Geometry: final body of the model. Coordinates: model frame, mm. A direction names the side the tool comes from. Round coordinates to 2 decimals unless told otherwise and drop trailing zeros. Write each loop counter-clockwise with the first axis right and the second up, starting at its lowest first coordinate (ties: lowest second). Pieces come first, ordered by that corner, then holes.
from build123d import *

# Parameters (mm, degrees)
ESQUISSE1_W             = 165.35
ESQUISSE1_H             = 84.146
BOSS_EXTRU_1_DEPTH      = 3.175
ESQUISSE2_W             = 3.175
ESQUISSE2_H             = 32.073
ENL_V_MAT_EXTRU_1_DEPTH = 93.819036727
ESQUISSE3_W             = 20
ESQUISSE3_H             = 3.175
ENL_V_MAT_EXTRU_2_DEPTH = 93.819036727


with BuildPart() as part:
    # Esquisse1 → Boss.-Extru.1 (new body)
    with BuildSketch(Plane.XY):
        Rectangle(ESQUISSE1_W, ESQUISSE1_H)
    extrude(amount=BOSS_EXTRU_1_DEPTH)

    # Esquisse2 → Enlèv. mat.-Extru.1 (cut, through all)
    with BuildSketch(Plane.XY.offset(3.175)):
        with Locations((-81.0875, -26.0365)):
            Rectangle(ESQUISSE2_W, ESQUISSE2_H)
        with Locations((-81.0875, 26.0365)):
            Rectangle(ESQUISSE2_W, ESQUISSE2_H)
    enl_v_mat_extru_1 = extrude(amount=-ENL_V_MAT_EXTRU_1_DEPTH, mode=Mode.SUBTRACT)

    # Symétrie1: Enlèv. mat.-Extru.1 across plane
    add(enl_v_mat_extru_1.mirror(Plane(origin=(0, 0, 0), x_dir=(0, 0, 1), z_dir=(1, 0, 0))), mode=Mode.SUBTRACT)

    # Esquisse3 → Enlèv. mat.-Extru.2 (cut, through all)
    with BuildSketch(Plane.XY.offset(3.175)):
        with Locations((0, -40.4855)):
            Rectangle(ESQUISSE3_W, ESQUISSE3_H)
        with Locations((40, -40.4855)):
            Rectangle(ESQUISSE3_W, ESQUISSE3_H)
        with Locations((-40, -40.4855)):
            Rectangle(ESQUISSE3_W, ESQUISSE3_H)
    enl_v_mat_extru_2 = extrude(amount=-ENL_V_MAT_EXTRU_2_DEPTH, mode=Mode.SUBTRACT)

    # Symétrie2: Enlèv. mat.-Extru.2 across plane
    add(enl_v_mat_extru_2.mirror(Plane.ZX), mode=Mode.SUBTRACT)


solid = part.part
1) Draft query along X for faces 4 (the flat face through (20, -42.073, 2)), 5 (the flat face through (-82.675, 0, 2)), 6 (the flat face through (-50, -41, 2)). Return one class per face: pulls with the +X half, pulls with the -X half, needs draft (parallel to the pull), parting line crosses it, or undercut.
2) First-contact query: P1, Ø1, axis at x = -40.5, y = -23, coming from the -Z side; P2, Ø1, axis at x = -44, z = 1, coming from the +Y side; P3, Ø1, axis at x = 36.5, z = 2, coming from the -Y side; P4, Ø1.6, axis at y = -40.5, z = 2, coming from the +X side. Flat tips, straight axial feed; report the tip coordinate or a pass-through.
3) Reachability of faces 1 (the flat face through (-40, 38.898, 2)), 2 (the flat face through (-79.5, 26, 2)), 3 (the flat face through (10, -41, 2)) from +Z, -Z, +X, -X, +Y, -Y: full face, straight path, thin tool, end or side. Return the list, or none.
4) Section A-A on y = -34. Output: boundary loops of the cut face in (x, z) (3 decimals), plus the area to 3 significant figures.
5) Line query: probe 1 along Y at (x, z) = (30.5, 2); probe 2 along X at (y, z) = (17.5, 0.7). Output: solid intervals per line, ascending.
6) Section B-B on x = 3. Output: boundary loops of the cut face in (y, z) (3 decimals).
Filled in:
1. face 4: needs draft
1. face 5: pulls with the -X half
1. face 6: undercut
2. P1: stops at z = 0
2. P2: stops at y = 38.9
2. P3: stops at y = -38.9
2. P4: stops at x = 79.5
3. face 1: +Z, -Z, +Y
3. face 2: +Z, -Z, -X, +Y
3. face 3: +Z, -Z, -Y
4. outline: (-79.5, 0) - (79.5, 0) - (79.5, 3.175) - (-79.5, 3.175) - close
4. area: 505 mm2
5. probe 1: y = -38.9 to 38.9
5. probe 2: x = -79.5 to 79.5
6. outline: (-38.898, 0) - (38.898, 0) - (38.898, 3.175) - (-38.898, 3.175) - close
